Source: CAD feature listing. Evaluate the final solid. Frame: model axes, mm. A direction names the side the tool comes from. Give positions to 0.01 mm unless a question says otherwise; leave off trailing zeros. Order: outer loops, then holes, each group sorted by start corner. A loop starts at its lowest first (then second) coordinate and runs counter-clockwise, first axis right, second up.
Autodesk Inventor part; units mm, degrees
ref_plane "Work Plane1" through (-17.3121, -15, 70.1) normal (0, 0, 1) x (1, 0, 0)
ref_plane "YZ Plane" through (0, 0, 0) normal (1, 0, 0) x (0, 1, 0)
ref_plane "XZ Plane" through (0, 0, 0) normal (0, 1, 0) x (-1, 0, 0)
sketch "Sketch1" plane through (0, 0, 0) normal (0, 0, 1) x (1, 0, 0)
  line L0 (-100, 100) -> (100, 100)
  line L1 (100, 100) -> (100, -100)
  line L2 (100, -100) -> (-100, -100)
  line L3 (-100, -100) -> (-100, 100)
  line L4 (-100, 100) -> (100, -100) construction
  line L5 (100, 100) -> (-100, -100) construction
  point P0 (0, 0)
  dimension "d0" = 200
  dimension "d1" = 200
extrude "Extrusion1" add sketch "Sketch1" along normal blind 5
ref_plane "Work Plane1" through (-17.3121, -15, 70.1) normal (0, 0, 1) x (1, 0, 0)
sketch "Sketch3" plane through (0, 0, 5) normal (0, 0, 1) x (1, 0, 0)
  line L0 (-13.3095, -15) -> (-13.3095, -20.1)
  line L1 (-13.3095, -14.5) -> (-18.3095, -14.5)
  line L2 (20.6905, -15) -> (20.6905, -20.1)
  line L3 (25.6905, -14.5) -> (20.6905, -14.5)
  line L4 (-13.3095, 20.1) -> (-13.3095, 15)
  line L5 (-18.3095, 14.5) -> (-13.3095, 14.5)
  line L6 (20.6905, 20.1) -> (20.6905, 15)
  line L7 (25.6905, 14.5) -> (20.6905, 14.5)
  line L8 (20.6905, -15) -> (25.6905, -15)
  line L9 (25.6905, -15) -> (25.6905, -20)
  line L10 (25.6905, -20) -> (20.6905, -20)
  line L11 (20.6905, -20) -> (20.6905, -15)
  line L12 (-13.3095, -20.1) -> (-28.3095, -20.1)
  line L13 (-28.3095, -20.1) -> (-28.3095, -15.1)
  line L14 (-28.3095, -15.1) -> (-13.3095, -15.1)
  line L15 (-13.3095, -15.1) -> (-13.3095, -20.1)
  line L16 (-13.3095, 20.1) -> (-28.3095, 20.1)
  line L17 (-28.3095, 20.1) -> (-28.3095, 15.1)
  line L18 (-28.3095, 15.1) -> (-13.3095, 15.1)
  line L19 (-13.3095, 15.1) -> (-13.3095, 20.1)
  line L20 (20.6905, 20.1) -> (25.6905, 20.1)
  line L21 (25.6905, 20.1) -> (25.6905, 15.1)
  line L22 (25.6905, 15.1) -> (20.6905, 15.1)
  line L23 (20.6905, 15.1) -> (20.6905, 20.1)
  point P0 (0, 0)
extrude "Extrusion2" add sketch "Sketch3" along normal up to surface (65.1 mm away)
chamfer "Chamfer1" distance 65.1 angle 45 5 edges at (-20.8095, 20.1, 5) (23.1905, 20.1, 5) (-28.3095, -20.1, 37.55) (-20.8095, -20.1, 5) (23.1905, -20, 5)
sketch "Sketch4" plane through (-28.3095, 15.1, 5) normal (-1, 0, 0) x (0, 0, 1)
  line L0 (0, 0) -> (65.1, 0)
  line L1 (65.1, 0) -> (40.1, 0)
  line L2 (65.1, 0) -> (90.1, 0) construction
  line L3 (0, -30.2) -> (65.1, -30.2)
  line L4 (40.1, 0) -> (0, 0)
  line L5 (0, 0) -> (0, -30.2)
  line L6 (0, -30.2) -> (40.1, -30.2)
  line L7 (40.1, -30.2) -> (40.1, 0)
  point P0 (-5, -15.1)
  dimension "d17" = 25
  dimension "d18" = 180
extrude "Extrusion3" add sketch "Sketch4" against normal blind 5
properties part number "base"
1) Pull-direction query (Y, two-part tool) for faces 4 (the face through (23, -15, 37)), 5 (the face through (-20.7, 52.2, 38)), 6 (the face through (-13.31, 43, 30)); classes: +Y half, -Y half, draft (parallel to the pull), parting line (faces both ways), or undercut.
Checks:
face 4: undercut
face 5: +Y half
face 6: draft
2) Section query C-C on z = 12.5. Output: boundary loops of the cut face in (x, y), and give its area (3 significant figures).
Checks:
outline: (-28.31, -77.7) - (-13.31, -77.7) - (-13.31, -15.1) - (-23.31, -15.1) - (-23.31, 15.1) - (-13.31, 15.1) - (-13.31, 77.7) - (-28.31, 77.7) - close; (20.69, -77.6) - (25.69, -77.6) - (25.69, -15) - (20.69, -15) - close; (20.69, 15.1) - (25.69, 15.1) - (25.69, 77.7) - (20.69, 77.7) - close
area: 2,650 mm2
3) Ray query, L1, parallel to X at y = -34, z = 18; L2, parallel to Z at x = 54, y = -73.5; L3, parallel to X at y = 11, z = 29.5. Return the intervals inside material, ascending.
Checks:
L1: x = -28.31 to -13.31, 20.69 to 25.69
L2: z = 0 to 5
L3: x = -28.31 to -23.31
4) Reachability of faces 1 (the face through (20.69, 43, 30)), 2 (the face through (-28.31, 1, 30)), 3 (the face through (25.69, 43, 30)) from +Z, -Z, +X, -X, +Y, -Y: full face, straight path, thin tool, end or side. Return the list, or none.
Checks:
face 1: +Z, +Y, -Y
face 2: +Z, -X, +Y, -Y
face 3: +Z, +X, +Y, -Y
5) Section query D-D on x = -59. Output: boundary loops of the cut face in (y, z).
Checks:
outline: (-100, 0) - (100, 0) - (100, 5) - (-100, 5) - close
6) Section query A-A on y = -7.5. Output: boundary loops of the cut face in (x, z).
Checks:
outline: (-100, 0) - (100, 0) - (100, 5) - (-23.31, 5) - (-23.31, 45.1) - (-28.31, 45.1) - (-28.31, 5) - (-100, 5) - close
7) First-contact query: pin 1 Ø24 at (y, z) = (0.5, 29.5) entering from +X; pin 2 Ø19.5 at (y, z) = (18, 45) entering from -X; pin 3 Ø1.5 at (x, y) = (73, -39) entering from -Z; pin 4 Ø5 at (y, z) = (13.5, 36.5) entering from +X. Flat tips, straight axial feed; report the tip coordinate or a pass-through.
Checks:
pin 1: stops at x = -23.31
pin 2: stops at x = -28.31
pin 3: stops at z = 0
pin 4: stops at x = 25.69
8) Section query B-B on z = 55. Output: boundary loops of the cut face in (x, y), and give its area (3 significant figures).
Checks:
outline: (-28.31, -35.2) - (-13.31, -35.2) - (-13.31, -15.1) - (-28.31, -15.1) - close; (-28.31, 15.1) - (-13.31, 15.1) - (-13.31, 35.2) - (-28.31, 35.2) - close; (20.69, -35.1) - (25.69, -35.1) - (25.69, -15) - (20.69, -15) - close; (20.69, 15.1) - (25.69, 15.1) - (25.69, 35.2) - (20.69, 35.2) - close
area: 804 mm2
